```python
from build123d import *

# Parameters (mm, degrees)
SKETCH1_R           = 1.75
BOSS_EXTRUDE1_DEPTH = 7
BOSS_EXTRUDE2_START = 7
SKETCH1_4_R         = 4
BOSS_EXTRUDE2_DEPTH = 7


with BuildPart() as part:
    # Sketch1 → Boss-Extrude1 (new body)
    with BuildSketch(Plane(origin=(0, 0, 0), x_dir=(0, 0, -1), z_dir=(1, 0, 0))):
        Polygon((-5, 11), (-10, 6), (-10, -6), (-5, -11), (30, -11), (30, -9), (90, -9), (90, 11), align=None)
        with Locations((34, 7)):
            Circle(SKETCH1_R, mode=Mode.SUBTRACT)
        with Locations((34, -5)):
            Circle(SKETCH1_R, mode=Mode.SUBTRACT)
        with BuildLine():
            Line((45, 6.75), (47, 6.75))
            ThreePointArc((47, 6.75), (48.75, 5), (47, 3.25))
            Line((47, 3.25), (45, 3.25))
            ThreePointArc((45, 3.25), (43.25, 5), (45, 6.75))
        make_face(mode=Mode.SUBTRACT)
        with BuildLine():
            Line((64, -3.25), (66, -3.25))
            ThreePointArc((66, -3.25), (67.75, -5), (66, -6.75))
            Line((66, -6.75), (64, -6.75))
            ThreePointArc((64, -6.75), (62.25, -5), (64, -3.25))
        make_face(mode=Mode.SUBTRACT)
        with BuildLine():
            Line((85, 3.25), (83, 3.25))
            ThreePointArc((83, 3.25), (81.25, 5), (83, 6.75))
            Line((83, 6.75), (85, 6.75))
            ThreePointArc((85, 6.75), (86.75, 5), (85, 3.25))
        make_face(mode=Mode.SUBTRACT)
    extrude(amount=BOSS_EXTRUDE1_DEPTH)

    # Sketch1<4> → Boss-Extrude2 (add)
    with BuildSketch(Plane(origin=(0, 0, 0), x_dir=(0, 0, -1), z_dir=(1, 0, 0)).offset(BOSS_EXTRUDE2_START)):
        Circle(SKETCH1_4_R)
    extrude(amount=BOSS_EXTRUDE2_DEPTH)


solid = part.part
```
Read the model definition and answer for the solid it produces. Units are mm, in the model's axes. A direction names the side the tool comes from. Round coordinates to 2 decimals unless told otherwise and drop trailing zeros. Write each loop counter-clockwise with the first axis right and the second up, starting at its lowest first coordinate (ties: lowest second). Pieces come first, ordered by that corner, then holes. Notation, with made-up numbers: (-33, 48.5) -> (-28, 48.5) arc R10 ccw to (-28, 63.5) -> close; hole circle Ø5 at (45.25, 79). An arc over 180 degrees is marked (long way). Answer in a Markdown table with one row per item. Add a question column.
1) Find section D-D, the plane z = -65. Determine the outline of the cut face in (x, y), and give its area (4 significant figures).
2) Given P1, Ø0.6, axis at x = 5, z = -46, coming from the -Y side; P2, Ø6, axis at x = 8, y = -6, coming from the -Z side; P3, Ø4, axis at x = 11, y = -4.5, coming from the +Z side; P4, Ø0.6, axis at x = 2.5, y = -10, coming from the -Z side, each flat-ended and moving along its own axis, determine where each tip first touches the part or whether it passes through.
3) Which of the six approach directions +Z, -Z, +X, -X, +Y, -Y give full straight-line access (tool end or side, diameter ignored) to faces 4 (the face through (3, 1, -90)), 5 (the face through (3.45, 5.04, -48.75))?
4) Determine the mould class of faces 1 (the face through (3, -3.25, -65)), 2 (the face through (7, 0, -39)), 3 (the face through (3, -11, -12)) for opening direction Y: pulls with the +Y half, pulls with the -Y half, needs draft (parallel to the pull), parting line crosses it, or undercut.
5) Find section B-B, the plane x = 4.5. Determine the outline of the cut face in (y, z).
6) Find section C-C, the plane y = 0. Determine the outline of the cut face in (x, z).
7) Find section A-A, the plane z = -34. Determine the outline of the cut face in (x, y).
8) Consider line 1 (Y direction, x = 3.5, z = -34); line 2 (Y direction, x = 4.25, z = -84.5); line 3 (X direction, y = 8, z = -45). Determine where each line is inside the solid, lowest interval first.
Findings below:
| question | item | result |
|---|---|---|
| 1 | outline | (0, -9) -> (7, -9) -> (7, -6.75) -> (0, -6.75) -> close; (0, -3.25) -> (7, -3.25) -> (7, 11) -> (0, 11) -> close |
| 1 | area | 115.5 mm² |
| 2 | P1 | y = -9 |
| 2 | P2 | z = -90 |
| 2 | P3 | z = 3.12 |
| 2 | P4 | z = -30 |
| 3 | face 4 | -Z, +X, -X, +Y, -Y |
| 3 | face 5 | +X, -X |
| 4 | face 1 | undercut |
| 4 | face 2 | needs draft |
| 4 | face 3 | pulls with the -Y half |
| 5 | outline | (-11, -30) -> (-9, -30) -> (-9, -90) -> (11, -90) -> (11, 5) -> (6, 10) -> (-6, 10) -> (-11, 5) -> close; hole (-6.75, -66) arc R1.75 ccw to (-3.25, -66) -> (-3.25, -64) arc R1.75 ccw to (-6.75, -64) -> close; hole circle Ø3.5 at (-5, -34); hole (3.25, -85) arc R1.75 ccw to (6.75, -85) -> (6.75, -83) arc R1.75 ccw to (3.25, -83) -> close; hole (3.25, -47) arc R1.75 ccw to (6.75, -47) -> (6.75, -45) arc R1.75 ccw to (3.25, -45) -> close; hole circle Ø3.5 at (7, -34) |
| 6 | outline | (0, -90) -> (7, -90) -> (7, -4) -> (14, -4) -> (14, 4) -> (7, 4) -> (7, 10) -> (0, 10) -> close |
| 7 | outline | (0, -9) -> (7, -9) -> (7, -6.75) -> (0, -6.75) -> close; (0, -3.25) -> (7, -3.25) -> (7, 5.25) -> (0, 5.25) -> close; (0, 8.75) -> (7, 8.75) -> (7, 11) -> (0, 11) -> close |
| 8 | line 1 | -9 to -6.75, -3.25 to 5.25, 8.75 to 11 |
| 8 | line 2 | -9 to 3.25, 6.75 to 11 |
| 8 | line 3 | 0 to 7 |
